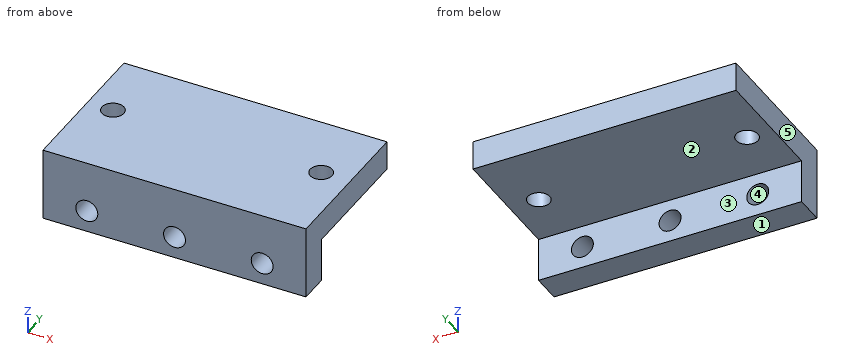
```python
from build123d import *

# Parameters (mm, degrees)
CROQUIS1_W              = 36
CROQUIS1_H              = 10
SALIENTE_EXTRUIR1_DEPTH = 7
CROQUIS3_W              = 36
CROQUIS3_H              = 4
SALIENTE_EXTRUIR2_DEPTH = 14
CROQUIS4_R              = 1.5
CORTAR_EXTRUIR1_DEPTH   = 10
CROQUIS5_R              = 1.5
CORTAR_EXTRUIR2_DEPTH   = 10
CROQUIS6_W              = 36
CROQUIS6_H              = 3
CORTAR_EXTRUIR3_DEPTH   = 6


with BuildPart() as part:
    # Croquis1 → Saliente-Extruir1 (new body)
    with BuildSketch(Plane(origin=(0, 0, 0), x_dir=(1, 0, 0), z_dir=(0, 1, 0))):
        with Locations((-18, -5)):
            Rectangle(CROQUIS1_W, CROQUIS1_H)
    extrude(amount=SALIENTE_EXTRUIR1_DEPTH)

    # Croquis3 → Saliente-Extruir2 (add)
    with BuildSketch(Plane(origin=(0, 7, 0), x_dir=(1, 0, 0), z_dir=(0, 1, 0))):
        with Locations((-18, -8)):
            Rectangle(CROQUIS3_W, CROQUIS3_H)
    extrude(amount=SALIENTE_EXTRUIR2_DEPTH)

    # Croquis4 → Cortar-Extruir1 (cut)
    with BuildSketch(Plane(origin=(0, 7, 0), x_dir=(1, 0, 0), z_dir=(0, 1, 0))):
        with Locations(Location((-30, -3, 0), (0, 0, 270))):
            Circle(CROQUIS4_R)
        with Locations(Location((-18, -3, 0), (0, 0, 270))):
            Circle(CROQUIS4_R)
        with Locations(Location((-6, -3, 0), (0, 0, 270))):
            Circle(CROQUIS4_R)
    extrude(amount=-CORTAR_EXTRUIR1_DEPTH, mode=Mode.SUBTRACT)

    # Croquis5 → Cortar-Extruir2 (cut)
    with BuildSketch(Plane.XY.offset(10)):
        with Locations((-32.5, 11.5)):
            Circle(CROQUIS5_R)
        with Locations((-4, 11.5)):
            Circle(CROQUIS5_R)
    extrude(amount=-CORTAR_EXTRUIR2_DEPTH, mode=Mode.SUBTRACT)

    # Croquis6 → Cortar-Extruir3 (cut)
    with BuildSketch(Plane(origin=(0, 0, 0), x_dir=(-1, 0, 0), z_dir=(0, 0, -1))):
        with Locations((18, 5.5)):
            Rectangle(CROQUIS6_W, CROQUIS6_H)
    extrude(amount=-CORTAR_EXTRUIR3_DEPTH, mode=Mode.SUBTRACT)


solid = part.part
```
Read the model definition and answer for the solid it produces. Units are mm, in the model's axes. Face numbers are marked on the shaded views. A direction names the side the tool comes from. Round coordinates to 2 decimals unless told otherwise and drop trailing zeros. Write each loop counter-clockwise with the first axis right and the second up, starting at its lowest first coordinate (ties: lowest second). Pieces come first, ordered by that corner, then holes. Notation, with made-up numbers: (-30, 71) -> (5, 71) arc R13 cw to (5, 85) -> close; hole circle Ø3 at (19, -9). An arc over 180 degrees is marked (long way). Answer in a Markdown table with one row per item. Add a question column.
1) Find section A-A, the plane y = 11.5. Determine the outline of the cut face in (x, z), and give its area (3 significant figures).
2) Consider line 1 (X direction, y = 2.6, z = 3); line 2 (X direction, y = 10.75, z = 8.75); line 3 (Y direction, x = -4, z = 9). Determine where each line is inside the solid, lowest interval first.
3) Which of the six approach directions +Z, -Z, +X, -X, +Y, -Y give full straight-line access (tool end or side, diameter ignored) to the marked faces 1 and 2?
4) Determine the mould class of the marked faces 3, 4 and 5 for opening direction X: pulls with the +X half, pulls with the -X half, needs draft (parallel to the pull), parting line crosses it, or undercut.
5) Find section C-C, the plane x = -32.5. Determine the outline of the cut face in (y, z), and give its area (3 significant figures).
6) Find section B-B, the plane z = 3. Determine the outline of the cut face in (x, y).
7) Given P1, Ø12, axis at x = -10, y = 15, coming from the -Z side; P2, Ø3.5, axis at x = -18, z = 3, coming from the +Y side, each flat-ended and moving along its own axis, determine where each tip first touches the part or whether it passes through.
8) Find section D-D, the plane z = 7. Determine the outline of the cut face in (x, y).
Findings below:
| question | item | result |
|---|---|---|
| 1 | outline | (-36, 6) -> (-34, 6) -> (-34, 10) -> (-36, 10) -> close; (-31, 6) -> (-5.5, 6) -> (-5.5, 10) -> (-31, 10) -> close; (-2.5, 6) -> (0, 6) -> (0, 10) -> (-2.5, 10) -> close |
| 1 | area | 120 mm² |
| 2 | line 1 | -36 to -31.5, -28.5 to -19.5, -16.5 to -7.5, -4.5 to 0 |
| 2 | line 2 | -36 to -33.8, -31.2 to -5.3, -2.7 to 0 |
| 2 | line 3 | 0 to 10, 13 to 21 |
| 3 | face 1 | -Z, +X, -X, +Y, -Y |
| 3 | face 2 | -Z, +X, -X, +Y |
| 4 | face 3 | needs draft |
| 4 | face 4 | undercut |
| 4 | face 5 | pulls with the -X half |
| 5 | outline | (0, 0) -> (4, 0) -> (4, 6) -> (10, 6) -> (10, 10) -> (0, 10) -> close; (13, 6) -> (21, 6) -> (21, 10) -> (13, 10) -> close |
| 5 | area | 96.0 mm² |
| 6 | outline | (-36, 0) -> (-31.5, 0) -> (-31.5, 4) -> (-36, 4) -> close; (-28.5, 0) -> (-19.5, 0) -> (-19.5, 4) -> (-28.5, 4) -> close; (-16.5, 0) -> (-7.5, 0) -> (-7.5, 4) -> (-16.5, 4) -> close; (-4.5, 0) -> (0, 0) -> (0, 4) -> (-4.5, 4) -> close |
| 7 | P1 | z = 6 |
| 7 | P2 | y = 4 |
| 8 | outline | (-36, 0) -> (0, 0) -> (0, 21) -> (-36, 21) -> close; hole circle Ø3 at (-32.5, 11.5); hole circle Ø3 at (-4, 11.5) |
